```python
from build123d import *

# Parameters (mm, degrees)
F0_W     = 190.5
F0_H     = 12.7
F1_DEPTH = 82.55
F2_R     = 17.4625
F3_DEPTH = 25.4
F4_W     = 25.4
F4_H     = 101.6
F5_DEPTH = 82.55
F7_DEPTH = 25.4
F8_R     = 20.6375
F9_DEPTH = 25.401


with BuildPart() as f1:
    # F0 (on Front) → F1 (new body)
    with BuildSketch(Plane.XZ):
        with Locations((95.25, 6.35)):
            Rectangle(F0_W, F0_H)
    extrude(amount=F1_DEPTH)

    # F2 (on face) → F3 (cut)
    with BuildSketch(Plane.XY.offset(12.7)):
        with Locations((76.2, -41.275)):
            Circle(F2_R)
        with Locations((152.4, -41.275)):
            Circle(F2_R)
    extrude(amount=-F3_DEPTH, mode=Mode.SUBTRACT)

    # F4 (on face) → F5 (join)
    with BuildSketch(Plane.XZ.offset(82.55)):
        with Locations((12.7, 63.5)):
            Rectangle(F4_W, F4_H)
    extrude(amount=-F5_DEPTH)

    # F6 (on face) → F7 (cut)
    with BuildSketch(Plane.YZ.offset(25.4)):
        with BuildLine():
            Line((-82.55, 114.3), (-82.55, 69.85))
            ThreePointArc((-82.55, 69.85), (-41.275, 111.125), (0, 69.85))
            Line((0, 69.85), (0, 114.3))
            Line((0, 114.3), (-82.55, 114.3))
        make_face()
    extrude(amount=-F7_DEPTH, mode=Mode.SUBTRACT)

    # F8 (on face) → F9 (cut, through all)
    with BuildSketch(Plane.YZ.offset(25.4)):
        with Locations((-41.275, 69.85)):
            Circle(F8_R)
    extrude(amount=-F9_DEPTH, mode=Mode.SUBTRACT)


solid = f1.part
```
CAD build for the part. Positions are in the model's coordinates, mm. A direction names the side the tool comes from. Coordinates: 2 decimals unless noted, no trailing zeros. Order: outer loops, then holes, each group sorted by start corner. A loop starts at its lowest first (then second) coordinate and runs counter-clockwise, first axis right, second up. Notation, with made-up numbers: M 29,-10 L 63,-10 A27 ccw 63,26 Z; hole C 46.25,23.25 d9. An arc over 180 degrees is marked long. Answer as CSV lines item,"result".
1) Mould opens along Y. For faces 1 (the flat face through (107, -41, 12.7)), 2 (the flat face through (60, -82.55, 12)), 3 (the cylindrical face through (12.878, -45.749, 49.703)) say: released by +Y, released by -Y, zero draft, split by the parting line, or undercut.
Verdict:
face 1,"zero draft"
face 2,"released by -Y"
face 3,"undercut"
2) Cut at B-B (y = -28). List the corners of the cut face in (x, z).
Verdict:
outline,"M 0,0 L 64.85,0 L 64.85,12.7 L 25.4,12.7 L 25.4,54.05 L 0,54.05 Z; M 0,85.65 L 25.4,85.65 L 25.4,108.93 L 0,108.93 Z; M 87.55,0 L 141.05,0 L 141.05,12.7 L 87.55,12.7 Z; M 163.75,0 L 190.5,0 L 190.5,12.7 L 163.75,12.7 Z"
3) Flat gauge pins, fed straight in: P1, Ø1.5, axis at y = -58.5, z = 94.5, coming from the +X side; P2, Ø21, axis at x = 152.4, y = -41.275, coming from the -Z side; P3, Ø12, axis at x = 99.5, y = -49.5, coming from the +Z side. Where does each tip first touch, or does it go through?
Verdict:
P1,"x = 25.4"
P2,"through"
P3,"z = 12.7"
4) Cut at A-A (x = 76.2). List the corners of the cut face in (y, z), then the cut area to 3 significant figures.
Verdict:
outline,"M -82.55,0 L -58.74,0 L -58.74,12.7 L -82.55,12.7 Z; M -23.81,0 L 0,0 L 0,12.7 L -23.81,12.7 Z"
area,"605 mm2"
5) Cut at C-C (z = 72). List the corners of the cut face in (x, y).
Verdict:
outline,"M 0,-82.49 L 25.4,-82.49 L 25.4,-61.8 L 0,-61.8 Z; M 0,-20.75 L 25.4,-20.75 L 25.4,-0.06 L 0,-0.06 Z"
6) Drill centre lines: L1, parallel to Y at x = 76, z = 3; L2, parallel to Z at x = 137, y = -30.5; L3, parallel to X at y = -57, z = 51. Where is each one in solid material? Low to high. Write a range as from..to.
Verdict:
L1,"-82.55..-58.74, -23.81..0"
L2,"0..12.7"
L3,"0..25.4"
7) 3-axis set-ups, long thin cutter, end or side, ignore diameter. For faces 4 (the flat face through (25.4, -51, 50)), 5 (the flat face through (60, 0, 12)): which of +Z, -Z, +X, -X, +Y, -Y reach the whole face in a straight line?
Verdict:
face 4,"+Z, +X, +Y, -Y"
face 5,"+Z, -Z, +X, -X, +Y"
8) Cut at D-D (z = 15). List the corners of the cut face in (x, y), then the cut area to 3 significant figures.
Verdict:
outline,"M 0,-82.55 L 25.4,-82.55 L 25.4,0 L 0,0 Z"
area,"2,100 mm2"
